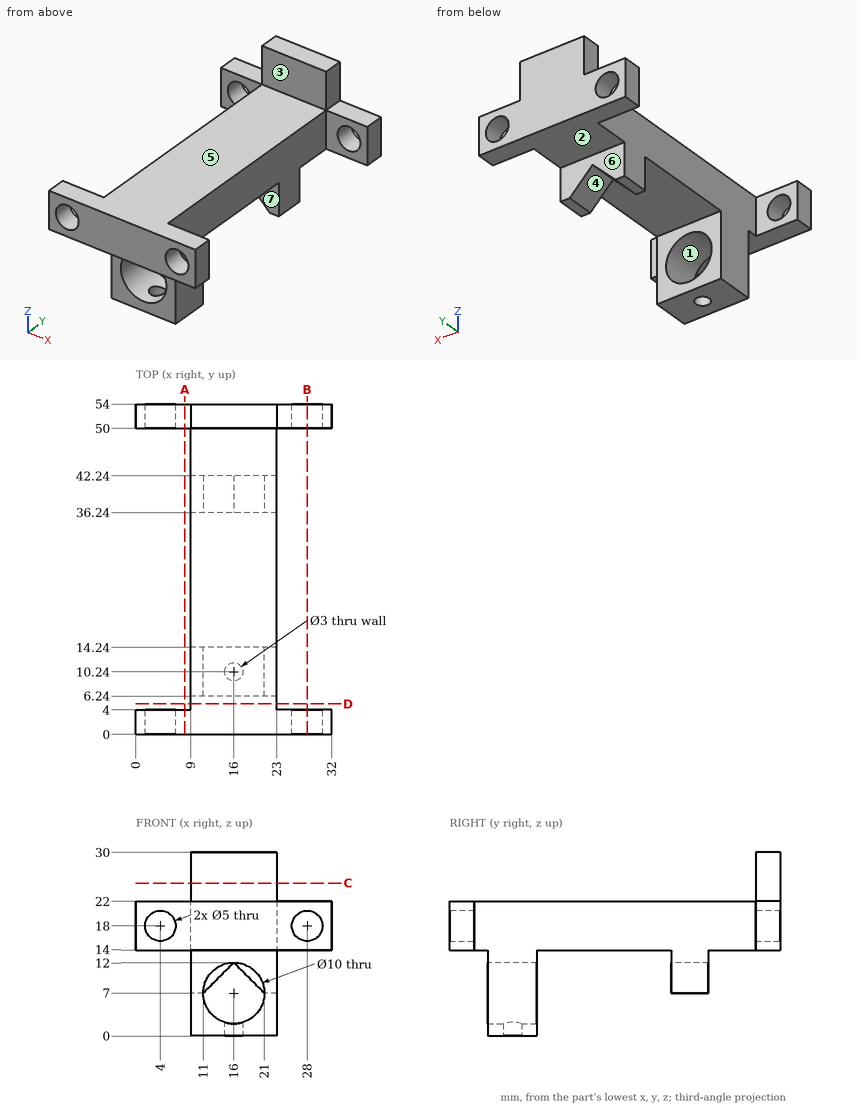
Verification items for this drawing (mm, ordinates from the low corner). A direction names the side the tool comes from. Give positions to 0.01 mm unless a question says otherwise; leave off trailing zeros. Loops run counter-clockwise (first coordinate to the right, second up) from the corner with the lowest first, then second, coordinate; pieces in that order, holes last. Notation, with made-up numbers: M 76,65 L 126,65 A30 cw 126,89 Z; hole C 82,-8 d11. An arc over 180 degrees is marked long. Return JSON: item names as keys, results as strings. Group by question number.
1. Cross-section at A-A on x = 8. Record the boundary of the cut face in (y, z).
2. Thickness scan on L1, parallel to X at y = 1.9, z = 18; L2, parallel to Y at x = 16, z = 1.05; L3, parallel to Y at x = 7, z = 17. Record the ranges inside material, lowest first.
3. Cross-section at C-C on z = 25. Record the boundary of the cut face in (x, y).
4. Go/stop test with flat-tipped pins: pin 1 (2 mm diameter, centred on y = 20, z = 21.5, fed in from -X); pin 2 (7.5 mm diameter, centred on x = 15, z = 10, fed in from +Y); pin 3 (2 mm diameter, centred on x = 8.5, y = 15.5, fed in from +Z); pin 4 (2 mm diameter, centred on x = 7, z = 8, fed in from +Y). Record where each tip stops, or that it passes through.
5. Cross-section at D-D on y = 5. Record the boundary of the cut face in (x, z).
6. Cross-section at B-B on x = 28. Record the boundary of the cut face in (y, z), plus the area to 3 significant figures.
7. Tool access check on the marked faces 1, 2, 3 and 4. Record the directions out of +Z, -Z, +X, -X, +Y, -Y that give a thin tool (end or side, any length) a straight path to the whole face; none if there is none.
8. Mould release check, pull along Y, two halves, no side actions. Record for the marked faces 5, 6 and 7: released by +Y, released by -Y, zero draft, split by the parting line, or undercut.
Return value:
{
 "1": {"outline": "M 0,14 L 4,14 L 4,22 L 0,22 Z; M 50,14 L 54,14 L 54,22 L 50,22 Z"},
 "2": {"L1": "0 to 1.5, 6.5 to 25.5, 30.5 to 32", "L2": "6.24 to 8.74, 11.74 to 14.24", "L3": "0 to 4, 50 to 54"},
 "3": {"outline": "M 9,50 L 23,50 L 23,54 L 9,54 Z"},
 "4": {"pin 1": "x = 9", "pin 2": "y = 42.24", "pin 3": "z = 22", "pin 4": "through"},
 "5": {"outline": "M 9,14 L 23,14 L 23,22 L 9,22 Z"},
 "6": {"outline": "M 0,14 L 4,14 L 4,15.5 L 0,15.5 Z; M 0,20.5 L 4,20.5 L 4,22 L 0,22 Z; M 50,14 L 54,14 L 54,15.5 L 50,15.5 Z; M 50,20.5 L 54,20.5 L 54,22 L 50,22 Z", "area": "24.0 mm^2"},
 "7": {"face 1": "-Y", "face 2": "-Z, +X, -X, +Y", "face 3": "+Z, +X, -X, -Y", "face 4": "-Z, +Y, -Y"},
 "8": {"face 5": "zero draft", "face 6": "released by +Y", "face 7": "undercut"}
}
